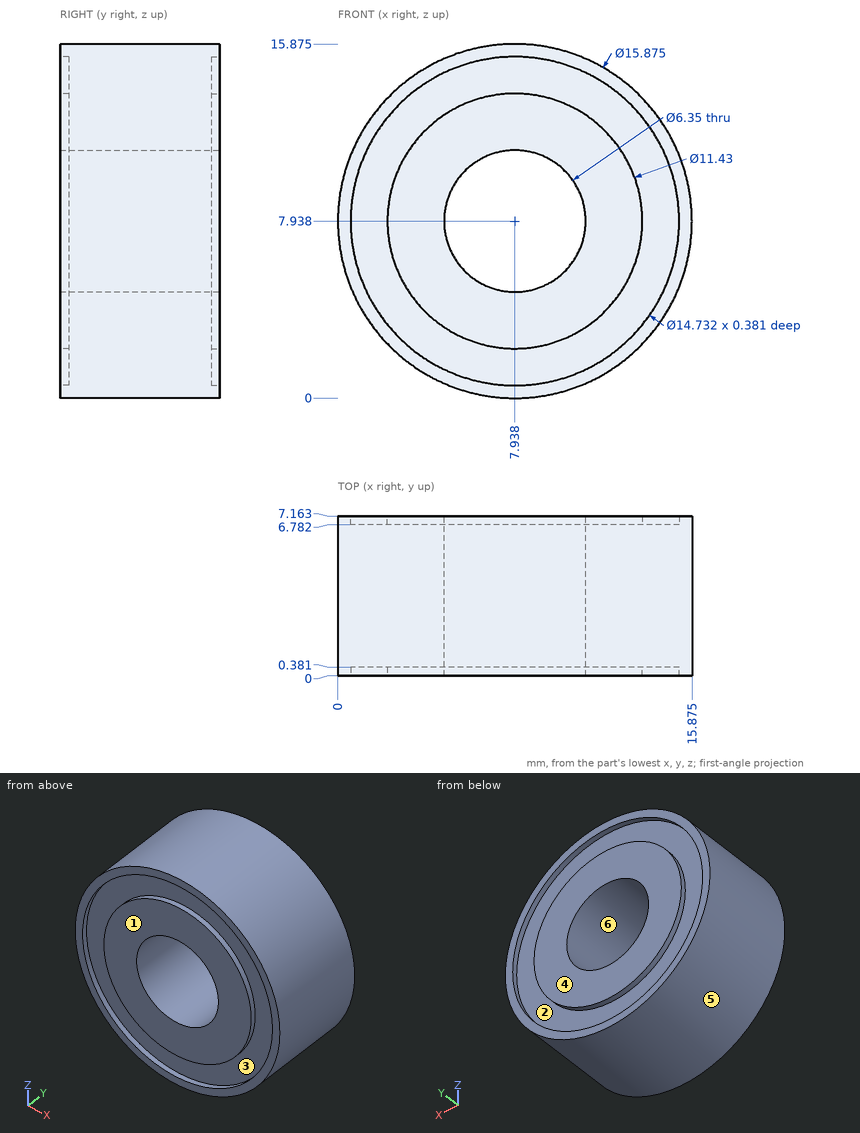
The figure shows three views and two pictorial views of one solid part (mm, origin at its lowest corner). Answer the questions. A direction names the side the tool comes from. Coordinates: 2 decimals unless noted, no trailing zeros. Use a Markdown table: item, result. Add a question column.
1) The mould has two halves that part along X. Classify the marked faces 3, 4, 5 and 6: released by +X, released by -X, zero draft, split by the parting line, or undercut.
2) Find the intervals of material crossed by line 1 (Z direction, x = 8, y = 5.5) (1 decimal); line 2 (X direction, y = 0.5, z = 8.75); line 3 (Z direction, x = 6.5, y = 4.75) (1 decimal), in increasing order.
3) Given pin 1 (2 mm diameter, centred on y = 1, z = 13.5, fed in from -X); pin 2 (1 mm diameter, centred on x = 13, y = 1.5, fed in from +Z); pin 3 (1 mm diameter, centred on y = 1, z = 2, fed in from +X), each flat-ended and moving along its own axis, determine where each tip first touches the part or whether it passes through.
4) For the marked faces 1 and 2, determine the directions among +Z, -Z, +X, -X, +Y, -Y from which every point of the face is accessible in a straight line to the end or side of a thin tool.
Here are the results:
| question | item | result |
|---|---|---|
| 1 | face 3 | undercut |
| 1 | face 4 | zero draft |
| 1 | face 5 | split by the parting line |
| 1 | face 6 | undercut |
| 2 | line 1 | z = 0 to 4.8, 11.1 to 15.9 |
| 2 | line 2 | x = 0.04 to 4.87, 11.01 to 15.83 |
| 2 | line 3 | z = 0.1 to 5.1, 10.8 to 15.7 |
| 3 | pin 1 | stops at x = 1.44 |
| 3 | pin 2 | stops at z = 14.43 |
| 3 | pin 3 | stops at x = 13.72 |
| 4 | face 1 | +Z, -Z, +X, -X, -Y |
| 4 | face 2 | +Y |
